Autodesk Inventor part; units mm, degrees
ref_plane "YZ Plane" through (0, 0, 0) normal (1, 0, 0) x (0, 1, 0)
ref_plane "XZ Plane" through (0, 0, 0) normal (0, 1, 0) x (-1, 0, 0)
ref_plane "XY Plane" through (0, 0, 0) normal (0, 0, 1) x (1, 0, 0)
sketch "Sketch2" plane through (0, 0, 0) normal (0, 0, 1) x (1, 0, 0)
  line L0 (-0.8337, 45.419) -> (-0.8337, -31.091)
  line L1 (-0.8337, -31.091) -> (14.1663, -18.5045)
  line L2 (14.1663, -18.5045) -> (14.1663, 23.419)
  line L3 (14.1663, 23.419) -> (23.1663, 23.419)
  line L4 (23.1663, 23.419) -> (23.1663, 28.419)
  line L5 (23.1663, 28.419) -> (16.1663, 28.419)
  line L6 (16.1663, 28.419) -> (16.1663, 40.419)
  line L7 (16.1663, 40.419) -> (25.1663, 40.419)
  line L8 (25.1663, 40.419) -> (25.1663, 45.419)
  line L9 (25.1663, 45.419) -> (-0.8337, 45.419)
  line L10 (16.1663, 28.419) -> (14.1663, 28.419) construction
  line L11 (1.3388, 42.919) -> (15.1663, 42.919)
  line L12 (15.1663, 42.919) -> (15.1663, 41.2824)
  line L13 (15.1663, 41.2824) -> (1.3388, 41.2824)
  line L14 (1.3388, 41.2824) -> (1.3388, 42.919)
  line L15 (11.0785, 23.419) -> (12.1663, 23.419)
  line L16 (12.1663, 23.419) -> (12.1663, -12.6156)
  line L17 (12.1663, -12.6156) -> (11.0785, -12.6156)
  line L18 (11.0785, -12.6156) -> (11.0785, 23.419)
  line L19 (2.2805, -14.4359) -> (12.1663, -14.4359)
  line L20 (12.1663, -14.4359) -> (12.1663, -16.121)
  line L21 (12.1663, -16.121) -> (2.2805, -16.121)
  line L22 (2.2805, -16.121) -> (2.2805, -14.4359)
  dimension "d17" = 2
  dimension "d18" = 7
  dimension "d19" = 9
  dimension "d20" = 5
  dimension "d21" = 5
  dimension "d22" = 15
  dimension "d23" = 12
  dimension "d24" = 2
  dimension "d25" = 46.9235
  dimension "d26" = 130
extrude "Extrusion1" add sketch "Sketch2" along normal blind 3 contours L9 L8 L7 L6 L5 L4 L3 L2 L1 L0 | L11 L12 L13 L14 | L15 L16 L17 L18 | L19 L20 L21 L22
properties part number "k2_t_side"
The model under review builds one solid part; all positions refer to its coordinate system, in mm. A direction names the side the tool comes from. Give positions to 0.01 mm unless a question says otherwise; leave off trailing zeros. Order: outer loops, then holes, each group sorted by start corner. A loop starts at its lowest first (then second) coordinate and runs counter-clockwise, first axis right, second up. Notation, with made-up numbers: M 19.5,7 L 66.5,7 A22 ccw 66.5,35 Z; hole C 39.25,-22 d6. An arc over 180 degrees is marked long. Answer in a Markdown table with one row per item. Add a question column.
1. For pin 1 Ø0.9 at (y, z) = (35, 2) entering from +X; pin 2 Ø0.9 at (x, z) = (18.5, 2) entering from -Y; pin 3 Ø1 at (y, z) = (19, 2.5) entering from +X, all flat-tipped, find the tip position at first contact; note any pin that passes through.
2. Add section B-B on y = 9. State the section outline as (x, z) points.
3. Mouldability with a two-part tool opening along Y and no side actions: class faces 1 (the flat face through (6.561, -24.886, 1.479)), 2 (the flat face through (21, 40.419, 1)), 3 (the flat face through (9, 16, 0)), 4 (the flat face through (20, 28.419, 1)) as released by +Y, released by -Y, zero draft, split by the parting line, or undercut.
4. Machinability: for faces 5 (the flat face through (19, 23.419, 1)), 6 (the flat face through (16.166, 34, 1)), 7 (the flat face through (12, 45.419, 1)), which of the approach directions +Z, -Z, +X, -X, +Y, -Y give a long, thin tool a straight path to every point of the face, cutting with its end or side? Answer none if there is none.
5. To check wall thickness, follow line 1 along Y through (x, z) = (23, 2.25); line 2 along X through (y, z) = (26.5, 2.7); line 3 along Y through (x, z) = (15, 1.3). State the ranges of each line that lie inside material, in increasing order.
6. Add section A-A on z = 2.2. State the section outline as (x, y) points, plus the area to 3 significant figures.
7. Add section C-C on x = 9.5. State the section outline as (y, z) points, plus the area to 3 significant figures.
The answers:
| question | item | result |
|---|---|---|
| 1 | pin 1 | x = 16.17 |
| 1 | pin 2 | y = 23.42 |
| 1 | pin 3 | x = 14.17 |
| 2 | outline | M -0.83,0 L 14.17,0 L 14.17,3 L -0.83,3 Z |
| 3 | face 1 | released by -Y |
| 3 | face 2 | undercut |
| 3 | face 3 | zero draft |
| 3 | face 4 | undercut |
| 4 | face 5 | +Z, -Z, +X, -Y |
| 4 | face 6 | +Z, -Z, +X |
| 4 | face 7 | +Z, -Z, +X, -X, +Y |
| 5 | line 1 | 23.42 to 28.42, 40.42 to 45.42 |
| 5 | line 2 | -0.83 to 23.17 |
| 5 | line 3 | 23.42 to 45.42 |
| 6 | outline | M -0.83,-31.09 L 14.17,-18.5 L 14.17,23.42 L 23.17,23.42 L 23.17,28.42 L 16.17,28.42 L 16.17,40.42 L 25.17,40.42 L 25.17,45.42 L -0.83,45.42 Z |
| 6 | area | 1,180 mm2 |
| 7 | outline | M -22.42,0 L 45.42,0 L 45.42,3 L -22.42,3 Z |
| 7 | area | 204 mm2 |
